from build123d import *

# Parameters (mm, degrees)
SKETCH6_R                 = 1.8542
CUT_EXTRUDE1_DEPTH        = 16.8115
F_6_32_TAPPED_HOLE1_D     = 2.7051
F_6_32_TAPPED_HOLE1_DEPTH = 4.318
F_6_32_TAPPED_HOLE1_TIP   = 0.81269403
CUT_EXTRUDE3_START        = -3.175
SKETCH12_R                = 15.08125
CUT_EXTRUDE3_DEPTH        = 13.6365
M16X1_5_TAPPED_HOLE1_D    = 14.5


with BuildPart() as part:
    # Sketch1 → Revolve1 (revolve)
    with BuildSketch(Plane.XY):
        Polygon((4.318, 50.673), (4.318, 47.371), (2.7305, 47.371), (2.7305, 44.2722), (-1.2065, 44.2722), (-1.2065, 47.371), (-2.794, 47.371), (-2.794, 44.2722), (-6.731, 44.2722), (-6.731, 47.371), (-8.3185, 47.371), (-8.3185, 41.0972), (0, 41.0972), (0, 0), (7.493, 0), (7.493, 50.673), align=None)
    revolve(axis=Axis((0, 0, 0), (1, 0, 0)))

    # Sketch6 → Cut-Extrude1 (cut, through all)
    with BuildSketch(Plane(origin=(7.493, 0, 0), x_dir=(0, 0, -1), z_dir=(1, 0, 0))):
        with Locations((22.225, 18.4785)):
            Circle(SKETCH6_R)
        with Locations((22.225, -18.4785)):
            Circle(SKETCH6_R)
        with BuildLine():
            Line((18.5547, 14.4272), (25.8953, 14.4272))
            ThreePointArc((25.8953, 14.4272), (26.344312806, 14.241212806), (26.5303, 13.7922))
            Line((26.5303, 13.7922), (26.5303, 11.7348))
            ThreePointArc((26.5303, 11.7348), (27.02874568, 10.53144568), (28.2321, 10.033))
            Line((28.2321, 10.033), (29.5275, 10.033))
            ThreePointArc((29.5275, 10.033), (30.73085432, 9.53455432), (31.2293, 8.3312))
            Line((31.2293, 8.3312), (31.2293, -8.3312))
            ThreePointArc((31.2293, -8.3312), (30.73085432, -9.53455432), (29.5275, -10.033))
            Line((29.5275, -10.033), (28.2321, -10.033))
            ThreePointArc((28.2321, -10.033), (27.02874568, -10.53144568), (26.5303, -11.7348))
            Line((26.5303, -11.7348), (26.5303, -13.7922))
            ThreePointArc((26.5303, -13.7922), (26.344312806, -14.241212806), (25.8953, -14.4272))
            Line((25.8953, -14.4272), (18.5547, -14.4272))
            ThreePointArc((18.5547, -14.4272), (18.105687194, -14.241212806), (17.9197, -13.7922))
            Line((17.9197, -13.7922), (17.9197, -11.7348))
            ThreePointArc((17.9197, -11.7348), (17.42125432, -10.53144568), (16.2179, -10.033))
            Line((16.2179, -10.033), (14.9225, -10.033))
            ThreePointArc((14.9225, -10.033), (13.71914568, -9.53455432), (13.2207, -8.3312))
            Line((13.2207, -8.3312), (13.2207, 8.3312))
            ThreePointArc((13.2207, 8.3312), (13.71914568, 9.53455432), (14.9225, 10.033))
            Line((14.9225, 10.033), (16.2179, 10.033))
            ThreePointArc((16.2179, 10.033), (17.42125432, 10.53144568), (17.9197, 11.7348))
            Line((17.9197, 11.7348), (17.9197, 13.7922))
            ThreePointArc((17.9197, 13.7922), (18.105687194, 14.241212806), (18.5547, 14.4272))
        make_face()
    extrude(amount=-CUT_EXTRUDE1_DEPTH, mode=Mode.SUBTRACT)

    # #6-32 Tapped Hole1
    with Locations(Plane.ZY):
        with Locations((0, 14.43482), (0, 0.54864)):
            Hole(F_6_32_TAPPED_HOLE1_D / 2, depth=F_6_32_TAPPED_HOLE1_DEPTH)
            with Locations((0, 0, -(F_6_32_TAPPED_HOLE1_DEPTH + F_6_32_TAPPED_HOLE1_TIP / 2))):  # 118° drill point
                Cone(0, F_6_32_TAPPED_HOLE1_D / 2, F_6_32_TAPPED_HOLE1_TIP, mode=Mode.SUBTRACT)

    # Sketch12 → Cut-Extrude3 (cut, through all)
    with BuildSketch(Plane(origin=(7.493, 0, 0), x_dir=(0, 0, -1), z_dir=(1, 0, 0)).offset(CUT_EXTRUDE3_START)):
        with Locations((0, -26.01595)):
            Circle(SKETCH12_R)
    extrude(amount=-CUT_EXTRUDE3_DEPTH, mode=Mode.SUBTRACT)

    # M16x1.5 Tapped Hole1 (through all)
    with Locations(Plane.ZY.offset(-4.318)):
        with Locations((0, -26.01595)):
            Hole(M16X1_5_TAPPED_HOLE1_D / 2)


solid = part.part
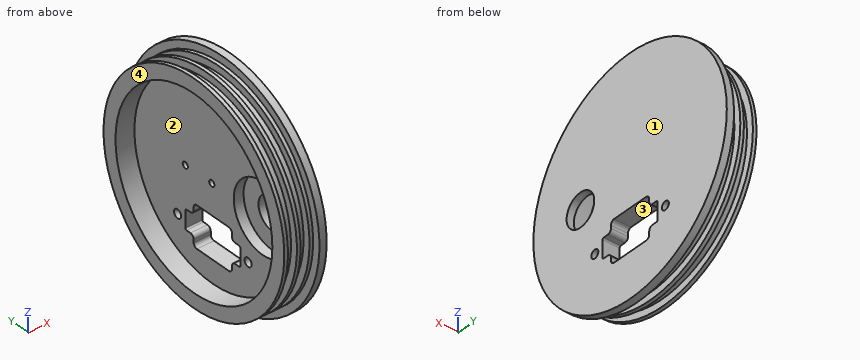
Geometry check sheet. Reference: the model listing, model coordinates, mm. Face numbers are marked on the shaded views. A direction names the side the tool comes from. Give positions to 0.01 mm unless a question says otherwise; leave off trailing zeros. Write each loop counter-clockwise with the first axis right and the second up, starting at its lowest first coordinate (ties: lowest second). Pieces come first, ordered by that corner, then holes. Notation, with made-up numbers: (89, 3) - (133, 3) arc R12 ccw to (133, 13) - close; hole circle Ø4 at (14, -29.5). An arc over 180 degrees is marked (long way). Put each result on its own line as item: value.
1. Sectioned sample at A-A, the plane z = 18. Enter the section's corners in (x, y), plus the area to 3 significant figures.
Ans:
outline: (-8.32, -43.82) - (-6.73, -43.82) - (-6.73, -40.45) - (-2.79, -40.45) - (-2.79, -43.82) - (-1.21, -43.82) - (-1.21, -40.45) - (2.73, -40.45) - (2.73, -43.82) - (4.32, -43.82) - (4.32, -47.37) - (7.49, -47.37) - (7.49, 47.37) - (4.32, 47.37) - (4.32, 43.82) - (2.73, 43.82) - (2.73, 40.45) - (-1.21, 40.45) - (-1.21, 43.82) - (-2.79, 43.82) - (-2.79, 40.45) - (-6.73, 40.45) - (-6.73, 43.82) - (-8.32, 43.82) - (-8.32, 36.95) - (0, 36.95) - (0, -36.95) - (-8.32, -36.95) - close
area: 740 mm²
2. Draft check along Z on the marked faces 3 and 4. Enter one of: +Z half, -Z half, draft (parallel to the pull), parting line (faces both ways), or undercut.
Ans:
face 3: undercut
face 4: draft
3. Sectioned sample at C-C, the plane z = -22.5. Give the number of separate pieces and of enclosed holes in the cut face, plus the area to 3 significant figures.
Ans:
separate pieces: 4
enclosed holes: 0
area: 442 mm²
4. Set-up check for the marked faces 1 and 2: record each of +Z, -Z, +X, -X, +Y, -Y from which the full face is reachable in a straight line by a thin tool's end or side.
Ans:
face 1: +Z, -Z, +X, +Y, -Y
face 2: -X
5. Thickness scan on line 1 (X direction, y = 21, z = -42); line 2 (Z direction, x = -2.5, y = 0); line 3 (Z direction, x = 5, y = -0.5). Record the ranges inside material, lowest first.
Ans:
line 1: x = -8.32 to -6.73, -2.79 to -1.21, 2.73 to 7.49
line 2: z = -47.37 to -41.1, 41.1 to 47.37
line 3: z = -50.67 to -31.23, -13.22 to 50.67
6. Sectioned sample at B-B, the plane y = 36. Enter the section's corners in (x, z).
Ans:
outline: (-8.32, -30.79) - (-6.73, -30.79) - (-6.73, -25.77) - (-2.79, -25.77) - (-2.79, -30.79) - (-1.21, -30.79) - (-1.21, -25.77) - (2.73, -25.77) - (2.73, -30.79) - (4.32, -30.79) - (4.32, -35.66) - (7.49, -35.66) - (7.49, 35.66) - (4.32, 35.66) - (4.32, 30.79) - (2.73, 30.79) - (2.73, 25.77) - (-1.21, 25.77) - (-1.21, 30.79) - (-2.79, 30.79) - (-2.79, 25.77) - (-6.73, 25.77) - (-6.73, 30.79) - (-8.32, 30.79) - (-8.32, 19.82) - (0, 19.82) - (0, -19.82) - (-8.32, -19.82) - close
7. Go/stop test with flat-tipped pins: pin 1 (24 mm diameter, centred on y = -23.5, z = 3, fed in from -X); pin 2 (1.6 mm diameter, centred on x = 4.5, y = -12.5, fed in from -Z); pin 3 (3 mm diameter, centred on x = -4.5, z = 10, fed in from -Y); pin 4 (13 mm diameter, centred on y = -26.02, z = 0, fed in from +X). Record where each tip stops, or that it passes through.
Ans:
pin 1: stops at x = 0
pin 2: stops at z = -49.3
pin 3: stops at y = -43.45
pin 4: passes through
